Geometry check sheet. Reference: the model listing, model coordinates, mm. A direction names the side the tool comes from. Give positions to 0.01 mm unless a question says otherwise; leave off trailing zeros.
1. Go/stop test with flat-tipped pins: pin 1 Ø4 at (y, z) = (19, 15.5) entering from +X; pin 2 Ø2 at (x, y) = (-1, 11) entering from -Z; pin 3 Ø10 at (x, y) = (-20, 12) entering from -Z. Record where each tip stops, or that it passes through.
2. Material ranges on L1, parallel to Y at x = 18, z = -27.5; L2, parallel to Y at x = -27, z = -4.5; L3, parallel to X at y = 19.75, z = -17, recorded low to high.
3. Tool access check on faces 1 (the flat face through (9.437, 16.501, -26.627)), 2 (the flat face through (-26.07, 8.2, 12.11)), 3 (the flat face through (0, 24, 0)), 4 (the flat face through (-27, 8.2, -9.87)), 5 (the flat face through (12.11, 8.2, 26.07)). Record the directions out of +Z, -Z, +X, -X, +Y, -Y that give a thin tool (end or side, any length) a straight path to the whole face; none if there is none.
Autodesk Inventor part; units mm, degrees
ref_plane "작업 평면24" through (-13.5, 24, -32.5919) normal (0, -0.622543, -0.7825856) x (1, 0, 0)
ref_plane "작업 평면26" through (32.5919, 0, -13.5) normal (0.5533716, 0.622543, -0.5533716) x (-0.7071068, 0, -0.7071068)
ref_plane "작업 평면27" through (0, 12, 0) normal (0, 1, 0) x (1, 0, 0)
sketch "스케치1" plane through (0, 0, 0) normal (0, 1, 0) x (-1, 0, 0)
  line L0 (-31.9919, 13.2515) -> (-13.2515, 31.9919)
  line L1 (-13.2515, 31.9919) -> (13.2515, 31.9919)
  line L2 (13.2515, 31.9919) -> (31.9919, 13.2515)
  line L3 (31.9919, 13.2515) -> (31.9919, -13.2515)
  line L4 (31.9919, -13.2515) -> (13.2515, -31.9919)
  line L5 (13.2515, -31.9919) -> (-13.2515, -31.9919)
  line L6 (-13.2515, -31.9919) -> (-31.9919, -13.2515)
  line L7 (-31.9919, -13.2515) -> (-31.9919, 13.2515)
  line L8 (-13.5, 32.5919) -> (13.5, 32.5919)
  line L9 (13.5, 32.5919) -> (32.5919, 13.5)
  line L10 (32.5919, 13.5) -> (32.5919, -13.5)
  line L11 (32.5919, -13.5) -> (13.5, -32.5919)
  line L12 (13.5, -32.5919) -> (-13.5, -32.5919)
  line L13 (-13.5, -32.5919) -> (-32.5919, -13.5)
  line L14 (-32.5919, -13.5) -> (-32.5919, 13.5)
  line L15 (-32.5919, 13.5) -> (-13.5, 32.5919)
  point P0 (0, 0)
  point P1 (0, 0)
  point P2 (0, 0)
  dimension "d2" = 0.6
  dimension "d118" = 27
extrude "돌출2" add sketch "스케치1" along normal blind 24 contours L0 L1 L2 L3 L4 L5 L6 L7 | L8 L9 L10 L11 L12 L13 L14 L15
ref_plane "작업 평면24" through (-13.5, 24, -32.5919) normal (0, -0.622543, -0.7825856) x (1, 0, 0)
sketch "스케치27" plane through (13.5, 0, -32.5919) normal (0, 0, -1) x (-1, 0, 0)
  line L0 (27, 24) -> (46.0919, 24)
  line L1 (0, 24) -> (27, 24)
  line L2 (27, 24) -> (0, 24)
  line L3 (0, 24) -> (-19.0919, 0)
  line L4 (-19.0919, 0) -> (27, 24)
  line L5 (0, 0) -> (0, 24)
  line L6 (0, 24) -> (0, 9.9411)
  point P0 (13.5, 0)
extrude "돌출22" cut sketch "스케치27" against normal up to surface surface through (-13.5, 24, -32.5919) normal (0, -0.622543, -0.7825856)
ref_plane "작업 평면26" through (32.5919, 0, -13.5) normal (0.5533716, 0.622543, -0.5533716) x (-0.7071068, 0, -0.7071068)
sketch "스케치28" plane through (13.5, 0, -32.5919) normal (0.7071068, 0, -0.7071068) x (-0.7071068, 0, -0.7071068)
  line L0 (-27.3314, 0) -> (-27.3314, 12)
  line L1 (19.0919, 0) -> (0, 0)
  line L2 (-27, 0) -> (0, 0)
  line L3 (19.0919, 0) -> (19.0919, 24)
  line L4 (0, 0) -> (19.0919, 24)
  line L5 (19.0919, 24) -> (-27, 0)
  point P0 (-13.5, 0)
  point P1 (-27.3314, 12)
extrude "돌출23" cut sketch "스케치28" against normal up to surface contours L2 L5 L4 surface through (32.5919, 0, -13.5) normal (0.5533716, 0.622543, -0.5533716)
pattern_circular "원형 패턴5" count 8 over 360 about axis through (0, -10, 0) along (0, 1, 0) of "돌출23", "돌출22"
ref_plane "작업 평면27" through (0, 12, 0) normal (0, 1, 0) x (1, 0, 0)
properties part number "팔각형 OV-PAM 층 한개"
Result:
1. pin 1: stops at x = 30.21
1. pin 2: stops at z = -31.97
1. pin 3: stops at z = -26.96
2. L1: y = 0 to 0.53, 17.6 to 18.34, 23.47 to 24
2. L2: y = 0 to 12.97, 16.97 to 24
2. L3: x = -24.31 to 24.31
3. face 1: -Z, +X
3. face 2: +Z, -X
3. face 3: +Z, -Z, +X, -X, +Y
3. face 4: -Z, -X
3. face 5: +Z, +X
